Source: three-view drawing plus pictorial views. Frame: mm from the lowest corner of the part. A direction names the side the tool comes from. Give positions to 0.01 mm unless a question says otherwise; leave off trailing zeros. Order: outer loops, then holes, each group sorted by start corner. A loop starts at its lowest first (then second) coordinate and runs counter-clockwise, first axis right, second up.
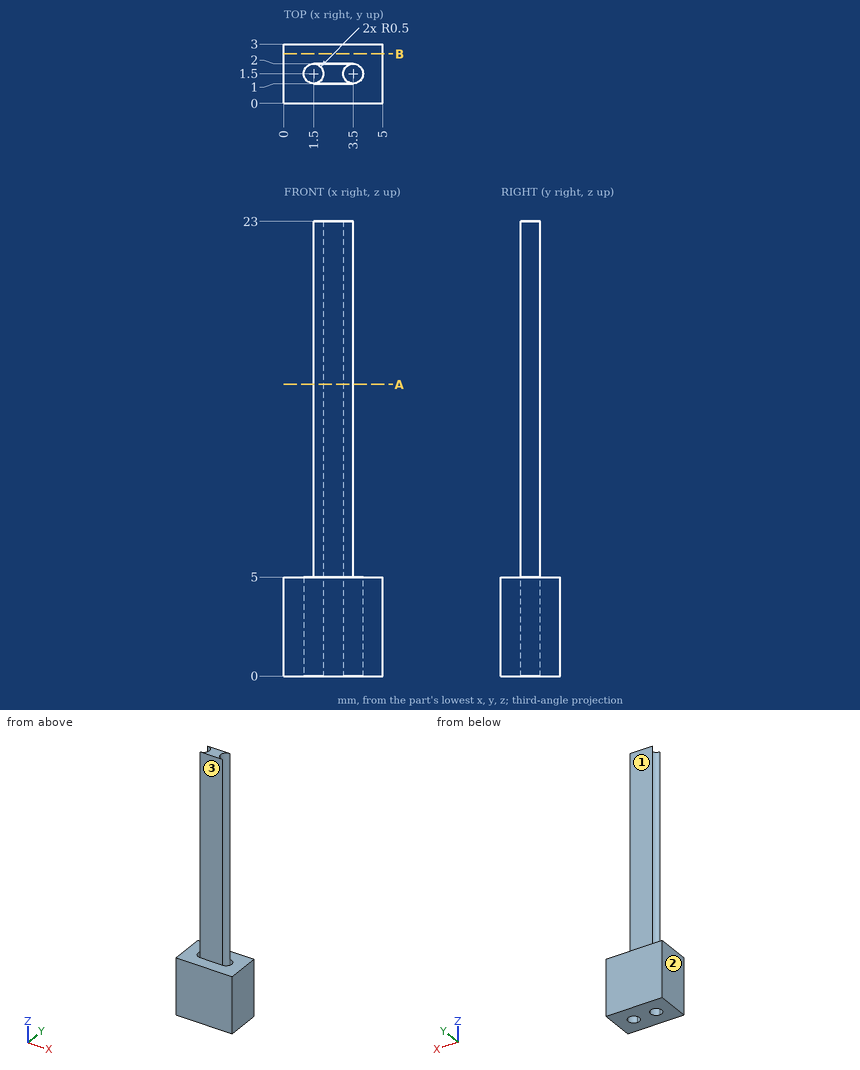
1) Section query A-A on z = 14.75. Output: boundary loops of the cut face in (x, y), and give its area (3 significant figures).
Checks:
outline: (1.5, 1) - (3.5, 1) arc R0.5 cw to (3, 1.5) arc R0.5 cw to (3.5, 2) - (1.5, 2) arc R0.5 cw to (2, 1.5) arc R0.5 cw to start
area: 1.21 mm2
2) First-contact query: pin 1 Ø0.6 at (x, z) = (2.5, 18) entering from -Y; pin 2 Ø0.6 at (x, z) = (2, 13.5) entering from +Y. Flat tips, straight axial feed; report the tip coordinate or a pass-through.
Checks:
pin 1: stops at y = 1
pin 2: stops at y = 2
3) Reachability of the marked faces 1, 2 and 3 from +Z, -Z, +X, -X, +Y, -Y: full face, straight path, thin tool, end or side. Return the list, or none.
Checks:
face 1: +Z, +X, -X, +Y
face 2: +Z, -Z, -X, +Y, -Y
face 3: +Z, +X, -X, -Y
4) Section query B-B on y = 2.5. Output: boundary loops of the cut face in (x, z).
Checks:
outline: (0, 0) - (5, 0) - (5, 5) - (0, 5) - close
5) Ray query, L1, parallel to X at y = 1.6, z = 3.75; L2, parallel to Z at x = 0.5, y = 2.7; L3, parallel to Y at x = 2.85, z = 8.75. Return the intervals inside material, ascending.
Checks:
L1: x = 0 to 1.01, 1.99 to 3.01, 3.99 to 5
L2: z = 0 to 5
L3: y = 1 to 2
